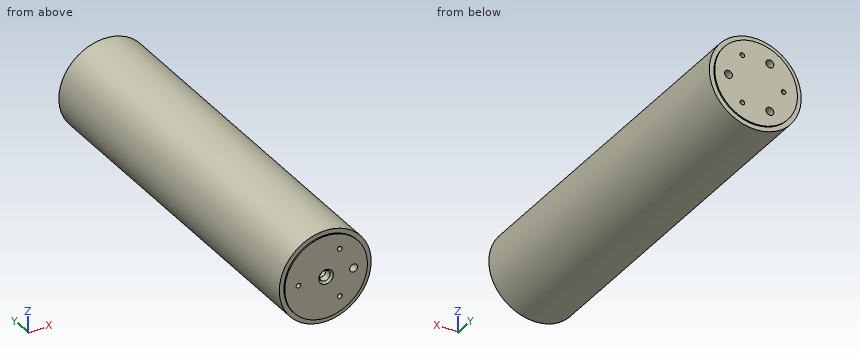
from build123d import *

# Parameters (mm, degrees)
SKETCH_5_R          = 5.7
SKETCH_5_R_2        = 4.28
CUT_EXTRUDE_4_DEPTH = 33
SKETCH_6_R          = 2.5
CUT_EXTRUDE_5_DEPTH = 5
CHAMFER_2_SIZE      = 2.2
EXTRUDE_START       = 1.5
SKETCH_7_R          = 45
EXTRUDE_1_DEPTH     = 1.5
CUT_EXTRUDE_START   = -5
SKETCH_8_R          = 2.5
CUT_EXTRUDE_6_DEPTH = 5
CUT_EXTRUDE_START_2 = -85
SKETCH_9_R          = 4.28
CUT_EXTRUDE_7_DEPTH = 85


with BuildPart() as part:
    # Эскиз2 → Повернуть2 (revolve)
    with BuildSketch(Plane(origin=(0, 0, 0), x_dir=(0, 0, -1), z_dir=(1, 0, 0))):
        Polygon((45, 1.5), (50, 1.5), (50, 396.5), (0, 396.5), (0, 388.5), (48, 388.5), (48, 9.5), (0, 9.5), (0, 0), (45, 0), align=None)
    revolve(axis=Axis((0, 0, 0), (0, 1, 0)))

    # Эскиз5 → Вырез-Вытянуть4 (cut)
    with BuildSketch(Plane.XZ):
        with Locations(Location((0, 0, 0), (0, 0, 270))):
            Circle(SKETCH_5_R)
        with Locations(Location((30, 0, 0), (0, 0, 270))):
            Circle(SKETCH_5_R_2)
    extrude(amount=-CUT_EXTRUDE_4_DEPTH, mode=Mode.SUBTRACT)

    # Эскиз6 → Вырез-Вытянуть5 (cut)
    with BuildSketch(Plane.XZ):
        with Locations(Location((-30, 0, 0), (0, 0, 270))):
            Circle(SKETCH_6_R)
        with Locations(Location((15, 25.980762114, 0), (0, 0, 270))):
            Circle(SKETCH_6_R)
        with Locations(Location((15, -25.980762114, 0), (0, 0, 270))):
            Circle(SKETCH_6_R)
    extrude(amount=-CUT_EXTRUDE_5_DEPTH, mode=Mode.SUBTRACT)

    # Фаска2
    chamfer_2_edges = [part.edges().sort_by_distance(p)[0] for p in [
        (0, 0, 5.7),
    ]]
    chamfer(chamfer_2_edges, length=CHAMFER_2_SIZE)

    # Эскиз7 → Бобышка-Вытянуть1 (add)
    with BuildSketch(Plane(origin=(0, 396.5, 0), x_dir=(1, 0, 0), z_dir=(0, 1, 0)).offset(EXTRUDE_START)):
        with Locations(Location((0, 0, 0), (0, 0, 90))):
            Circle(SKETCH_7_R)
    extrude(amount=-EXTRUDE_1_DEPTH)

    # Эскиз8 → Вырез-Вытянуть6 (cut)
    with BuildSketch(Plane(origin=(0, 398, 0), x_dir=(1, 0, 0), z_dir=(0, 1, 0)).offset(CUT_EXTRUDE_START)):
        with Locations(Location((-30, 0, 0), (0, 0, 90))):
            Circle(SKETCH_8_R)
        with Locations(Location((15, 25.980762114, 0), (0, 0, 90))):
            Circle(SKETCH_8_R)
        with Locations(Location((15, -25.980762114, 0), (0, 0, 90))):
            Circle(SKETCH_8_R)
    extrude(amount=CUT_EXTRUDE_6_DEPTH, mode=Mode.SUBTRACT)

    # Эскиз9 → Вырез-Вытянуть7 (cut)
    with BuildSketch(Plane(origin=(0, 398, 0), x_dir=(1, 0, 0), z_dir=(0, 1, 0)).offset(CUT_EXTRUDE_START_2)):
        with Locations(Location((30, 0, 0), (0, 0, 90))):
            Circle(SKETCH_9_R)
        with Locations(Location((-15, -25.980762114, 0), (0, 0, 270))):
            Circle(SKETCH_9_R)
        with Locations(Location((-15, 25.980762114, 0), (0, 0, 270))):
            Circle(SKETCH_9_R)
    extrude(amount=CUT_EXTRUDE_7_DEPTH, mode=Mode.SUBTRACT)


solid = part.part
CAD build for the part. Positions are in the model's coordinates, mm. Coordinates: 2 decimals unless noted, no trailing zeros. Write each loop counter-clockwise with the first axis right and the second up, starting at its lowest first coordinate (ties: lowest second). Pieces come first, ordered by that corner, then holes. Notation, with made-up numbers: M -5,55.25 L 21,55.25 A19 cw 21,91.25 Z; hole C -24.5,-14 d6. An arc over 180 degrees is marked long. Answer as a JSON object with one key per item and string values. Group by question number.
1) Saw through at C-C (x = 0). Write the cut outline in (y, z).
2) Pin check, flat tips, straight feed: pin 1 Ø2.5 at (x, z) = (15.5, -27) entering from -Y; pin 2 Ø7.5 at (x, z) = (30, 0) entering from -Y; pin 3 Ø4 at (x, y) = (30.5, 296.5) entering from +Z; pin 4 Ø5 at (x, z) = (-15, 25.98) entering from +Y. Stop position of each tip, or through.
3) Saw through at D-D (z = 14). Write the cut outline in (x, y), plus the area to 3 significant figures.
4) Wall check: line 1 (Y direction, x = 11, z = -40.5); line 2 (Z direction, x = 0, y = 253); line 3 (Y direction, x = -32.5, z = 32). Give the ranges that are in metal, low to high. Write a range as from..to.
5) Saw through at B-B (y = 362). Write the cut outline in (x, z), plus the area to 3 significant figures.
6) Saw through at A-A (x = 30). Write the cut outline in (y, z), plus the area to 3 significant figures.
Values follow:
{
 "1": {"outline": "M 0,-45 L 1.5,-45 L 1.5,-50 L 396.5,-50 L 396.5,-45 L 398,-45 L 398,45 L 396.5,45 L 396.5,50 L 1.5,50 L 1.5,45 L 0,45 L 0,7.9 L 2.2,5.7 L 9.5,5.7 L 9.5,48 L 388.5,48 L 388.5,-48 L 9.5,-48 L 9.5,-5.7 L 2.2,-5.7 L 0,-7.9 Z"},
 "2": {"pin 1": "stops at y = 5", "pin 2": "passes through", "pin 3": "stops at z = 41.08", "pin 4": "stops at y = 9.5"},
 "3": {"outline": "M -48,1.5 L -42.77,1.5 L -42.77,0 L 42.77,0 L 42.77,1.5 L 48,1.5 L 48,396.5 L 42.77,396.5 L 42.77,398 L -42.77,398 L -42.77,396.5 L -48,396.5 Z; hole M -45.91,9.5 L 45.91,9.5 L 45.91,388.5 L -45.91,388.5 Z", "area": "3,370 mm2"},
 "4": {"line 1": "y = 0..9.5, 388.5..398", "line 2": "z = -50..-48, 48..50", "line 3": "y = 1.5..9.5, 388.5..396.5"},
 "5": {"outline": "C 0,0 d100; hole C 0,0 d96", "area": "616 mm2"},
 "6": {"outline": "M 0,-33.54 L 1.5,-33.54 L 1.5,-40 L 396.5,-40 L 396.5,-33.54 L 398,-33.54 L 398,-4.28 L 388.5,-4.28 L 388.5,-37.47 L 9.5,-37.47 L 9.5,-4.28 L 0,-4.28 Z; M 0,4.28 L 9.5,4.28 L 9.5,37.47 L 388.5,37.47 L 388.5,4.28 L 398,4.28 L 398,33.54 L 396.5,33.54 L 396.5,40 L 1.5,40 L 1.5,33.54 L 0,33.54 Z", "area": "3,240 mm2"}
}
